Model file for the job. Use its own axes, mm. A direction names the side the tool comes from. Coordinates: 2 decimals unless noted, no trailing zeros. Write each loop counter-clockwise with the first axis right and the second up, starting at its lowest first coordinate (ties: lowest second). Pieces come first, ordered by that corner, then holes. Notation, with made-up numbers: M 56,7 L 99,7 A21 cw 99,26 Z; hole C 77,67 d7. An arc over 180 degrees is marked long. Use CSV: the item, a comma, the result in double quotes. Start each with the question number.
from build123d import *

# Parameters (mm, degrees)
F1_DEPTH = 3.175
F3_DEPTH = 6.35


with BuildPart() as f1:
    # F0 (on Right) → F1 (new body)
    with BuildSketch(Plane.YZ):
        with BuildLine():
            ThreePointArc((11.2416642137, 13.194756409), (18.2070674879, 9.4741128861), (24.0282094439, 4.1379778313))
            Line((24.0282094439, 4.1379778313), (35.6114845565, 13.9572464754))
            ThreePointArc((35.6114845565, 13.9572464754), (24.8807782287, 23.2715946139), (11.8451676598, 28.9265036877))
            ThreePointArc((11.8451676598, 28.9265036877), (10.0327447326, 32.0278458379), (13.1340868829, 33.8402687651))
            ThreePointArc((13.1340868829, 33.8402687651), (27.588153444, 27.5700268215), (39.4865100795, 17.2421478736))
            Line((39.4865100795, 17.2421478736), (46.5087493001, 23.1949766478))
            ThreePointArc((46.5087493001, 23.1949766478), (0, 44.7400710849), (-46.5087493001, 23.1949766478))
            Line((-46.5087493001, 23.1949766478), (-39.4865100795, 17.2421478736))
            ThreePointArc((-39.4865100795, 17.2421478736), (-27.588153444, 27.5700268215), (-13.1340868829, 33.8402687651))
            ThreePointArc((-13.1340868829, 33.8402687651), (-10.0327447326, 32.0278458379), (-11.8451676598, 28.9265036877))
            ThreePointArc((-11.8451676598, 28.9265036877), (-24.8807782287, 23.2715946139), (-35.6114845565, 13.9572464754))
            Line((-35.6114845565, 13.9572464754), (-24.0282094439, 4.1379778313))
            ThreePointArc((-24.0282094439, 4.1379778313), (-18.2070674879, 9.4741128861), (-11.2416642137, 13.194756409))
            Line((-11.2416642137, 13.194756409), (-11.7119892349, 14.7131928424))
            Line((-11.7119892349, 14.7131928424), (-7.8299477766, 15.9156279202))
            Line((-7.8299477766, 15.9156279202), (-7.3596227555, 14.3971914867))
            ThreePointArc((-7.3596227555, 14.3971914867), (-4.7130812866, 14.9144174535), (-2.032, 15.2033942376))
            Line((-2.032, 15.2033942376), (-2.032, 16.7930026258))
            Line((-2.032, 16.7930026258), (2.032, 16.7930026258))
            Line((2.032, 16.7930026258), (2.032, 15.2033942376))
            ThreePointArc((2.032, 15.2033942376), (4.7130812866, 14.9144174535), (7.3596227555, 14.3971914867))
            Line((7.3596227555, 14.3971914867), (7.8299477766, 15.9156279202))
            Line((7.8299477766, 15.9156279202), (11.7119892349, 14.7131928424))
            Line((11.7119892349, 14.7131928424), (11.2416642137, 13.194756409))
        make_face()
    extrude(amount=F1_DEPTH)

    # F2 (on face) → F3 (join)
    with BuildSketch(Plane(origin=(0, 0, 0), x_dir=(0, -1, 0), z_dir=(-1, 0, 0))):
        with BuildLine():
            Line((-2.032, 16.7930026258), (2.032, 16.7930026258))
            Line((2.032, 16.7930026258), (2.032, 15.2690026258))
            Line((2.032, 15.2690026258), (2.032, 15.2033942376))
            ThreePointArc((2.032, 15.2033942376), (4.7130812866, 14.9144174535), (7.3596227555, 14.3971914867))
            Line((7.3596227555, 14.3971914867), (7.3790346224, 14.4598623733))
            Line((7.3790346224, 14.4598623733), (7.8299477766, 15.9156279202))
            Line((7.8299477766, 15.9156279202), (11.7119892349, 14.7131928424))
            Line((11.7119892349, 14.7131928424), (11.2610760807, 13.2574272956))
            Line((11.2610760807, 13.2574272956), (11.2416642137, 13.194756409))
            ThreePointArc((11.2416642137, 13.194756409), (18.2070674879, 9.4741128861), (24.0282094439, 4.1379778313))
            Line((24.0282094439, 4.1379778313), (35.6114845565, 13.9572464754))
            ThreePointArc((35.6114845565, 13.9572464754), (24.8807782287, 23.2715946139), (11.8451676598, 28.9265036877))
            ThreePointArc((11.8451676598, 28.9265036877), (10.0327447326, 32.0278458379), (13.1340868829, 33.8402687651))
            ThreePointArc((13.1340868829, 33.8402687651), (27.588153444, 27.5700268215), (39.4865100795, 17.2421478736))
            Line((39.4865100795, 17.2421478736), (46.5087493001, 23.1949766478))
            ThreePointArc((46.5087493001, 23.1949766478), (0, 44.7400710849), (-46.5087493001, 23.1949766478))
            Line((-46.5087493001, 23.1949766478), (-39.4865100795, 17.2421478736))
            ThreePointArc((-39.4865100795, 17.2421478736), (-27.588153444, 27.5700268215), (-13.1340868829, 33.8402687651))
            ThreePointArc((-13.1340868829, 33.8402687651), (-10.0327447326, 32.0278458379), (-11.8451676598, 28.9265036877))
            ThreePointArc((-11.8451676598, 28.9265036877), (-24.8807782287, 23.2715946139), (-35.6114845565, 13.9572464754))
            Line((-35.6114845565, 13.9572464754), (-24.0282094439, 4.1379778313))
            ThreePointArc((-24.0282094439, 4.1379778313), (-18.2070674879, 9.4741128861), (-11.2416642137, 13.194756409))
            Line((-11.2416642137, 13.194756409), (-11.2610760807, 13.2574272956))
            Line((-11.2610760807, 13.2574272956), (-11.7119892349, 14.7131928424))
            Line((-11.7119892349, 14.7131928424), (-7.8299477766, 15.9156279202))
            Line((-7.8299477766, 15.9156279202), (-7.3790346224, 14.4598623733))
            Line((-7.3790346224, 14.4598623733), (-7.3596227555, 14.3971914867))
            ThreePointArc((-7.3596227555, 14.3971914867), (-4.7130812866, 14.9144174535), (-2.032, 15.2033942376))
            Line((-2.032, 15.2033942376), (-2.032, 15.2690026258))
            Line((-2.032, 15.2690026258), (-2.032, 16.7930026258))
        make_face()
    extrude(amount=F3_DEPTH)


solid = f1.part
1) Band-saw the part on C-C on z = 10. List the corners of the cut face in (x, y) (3 decimals).
2) Band-saw the part on A-A on y = 31. List the corners of the cut face in (x, z) (3 decimals), then the cut area to 3 significant figures.
3) Two-plate mould, pull along Y, no slides. Class faces 4 (the face through (-6.35, 1, 25)), 5 (the face through (-1.52, -10.02, 31.97)), 6 (the face through (-1.521, 29.901, 9.116)), 7 (the face through (-1.52, -29.74, 8.98)): pulls with the +Y half, pulls with the -Y half, needs draft (parallel to the pull), parting line crosses it, or undercut.
4) Tool access for faces 1 (the face through (-1.5, 4.8, 14.9)), 2 (the face through (-1.52, -42.95, 20.18)), 3 (the face through (-1.521, -25.05, 23.165)): list every direction of +Z, -Z, +X, -X, +Y, -Y with a clear straight run to the whole face (end or side of a thin tool).
5) Drop flat-ended pins along their axis: P1, Ø0.8, axis at x = -3, z = 15.5, coming from the -Y side; P2, Ø1.7, axis at x = -4, z = 16, coming from the +Y side (3 decimals); P3, Ø3.5, axis at x = -3.5, y = -0.5, coming from the -Z side. Give the stop position or say it passes through.
6) Wall check: L1, parallel to Y at x = 0.5, z = 19.5; L2, parallel to Y at x = 0.25, z = 20; L3, parallel to Y at x = -4.5, z = 10. Give the ranges that are in metal, low to high. Write a range as [from, to].
7) Band-saw the part on D-D on x = 1.75. List the corners of the cut face in (y, z).
8) Band-saw the part on B-B on z = 21.5. List the corners of the cut face in (x, y) (3 decimals), then the cut area to 3 significant figures.
Findings below:
1,outline,"M -6.35,-30.943 L 3.175,-30.943 L 3.175,-17.441 L -6.35,-17.441 Z; M -6.35,17.441 L 3.175,17.441 L 3.175,30.943 L -6.35,30.943 Z"
2,outline,"M -6.35,10.048 L 3.175,10.048 L 3.175,18.676 L -6.35,18.676 Z; M -6.35,25.225 L 3.175,25.225 L 3.175,36.271 L -6.35,36.271 Z"
2,area,"187 mm2"
3,face 4,"needs draft"
3,face 5,"undercut"
3,face 6,"pulls with the +Y half"
3,face 7,"pulls with the -Y half"
4,face 1,"-Z, +X, -X"
4,face 2,"-Z, +X, -X, -Y"
4,face 3,"+X, -X"
5,P1,"stops at y = -34.61"
5,P2,"stops at y = 34.565"
5,P3,"stops at z = 15.19"
6,L1,"y = [-42.15, -37.46], [-30.05, 30.05], [37.46, 42.15]"
6,L2,"y = [-42.74, -36.97], [-29.44, 29.44], [36.97, 42.74]"
6,L3,"y = [-30.94, -17.44], [17.44, 30.94]"
7,outline,"M -46.51,23.19 L -39.49,17.24 A51.77 cw -13.13,33.84 A2.54 cw -11.85,28.93 A46.69 ccw -35.61,13.96 L -24.03,4.14 A31.5 cw -11.24,13.19 L -11.71,14.71 L -7.83,15.92 L -7.36,14.4 A31.5 cw -2.03,15.2 L -2.03,16.79 L 2.03,16.79 L 2.03,15.2 A31.5 cw 7.36,14.4 L 7.83,15.92 L 11.71,14.71 L 11.24,13.19 A31.5 cw 24.03,4.14 L 35.61,13.96 A46.69 ccw 11.85,28.93 A2.54 cw 13.13,33.84 A51.77 cw 39.49,17.24 L 46.51,23.19 A60.97 ccw Z"
8,outline,"M -6.35,-44.509 L 3.175,-44.509 L 3.175,-35.44 L -6.35,-35.44 Z; M -6.35,-27.493 L 3.175,-27.493 L 3.175,27.493 L -6.35,27.493 Z; M -6.35,35.44 L 3.175,35.44 L 3.175,44.509 L -6.35,44.509 Z"
8,area,"697 mm2"
